```python
from build123d import *

# Parameters (mm, degrees)
BOSS_EXTRUDE1_DEPTH = 10
SKETCH2_R           = 1.5
BOSS_EXTRUDE2_DEPTH = 8


with BuildPart() as part:
    # Sketch1 → Boss-Extrude1 (new body)
    with BuildSketch(Plane(origin=(0, 0, 0), x_dir=(1, 0, 0), z_dir=(0, 1, 0))):
        Polygon((3.175426481, 0), (1.58771324, 2.75), (-1.58771324, 2.75), (-3.175426481, 0), (-1.58771324, -2.75), (1.58771324, -2.75), align=None)
    extrude(amount=-BOSS_EXTRUDE1_DEPTH)

    # Sketch2 → Boss-Extrude2 (add)
    with BuildSketch(Plane(origin=(0, 0, 0), x_dir=(1, 0, 0), z_dir=(0, 1, 0))):
        with Locations(Location((0, 0, 0), (0, 0, 270))):
            Circle(SKETCH2_R)
    extrude(amount=BOSS_EXTRUDE2_DEPTH)


solid = part.part
```
Input: part model. Units: mm. Frame: model coordinates. A direction names the side the tool comes from. Coordinates: 2 decimals unless noted, no trailing zeros. Loops run counter-clockwise (first coordinate to the right, second up) from the corner with the lowest first, then second, coordinate; pieces in that order, holes last. Notation, with made-up numbers: (13, 41) - (64, 41) arc R10 ccw to (64, 50) - close; hole circle Ø4 at (61, 63). An arc over 180 degrees is marked (long way). Answer in a Markdown table with one row per item.
(1) Cut plane D-D on y = 6.75. Output: boundary loops of the cut face in (x, z), plus the area to 3 significant figures.
Model answer:
| item | result |
|---|---|
| outline | circle Ø3 at (0, 0) |
| area | 7.07 mm² |
(2) Cut plane A-A on y = -3. Output: boundary loops of the cut face in (x, z), plus the area to 3 significant figures.
Model answer:
| item | result |
|---|---|
| outline | (-3.18, 0) - (-1.59, -2.75) - (1.59, -2.75) - (3.18, 0) - (1.59, 2.75) - (-1.59, 2.75) - close |
| area | 26.2 mm² |
(3) Cut plane B-B on x = 0. Output: boundary loops of the cut face in (y, z).
Model answer:
| item | result |
|---|---|
| outline | (-10, -2.75) - (0, -2.75) - (0, -1.5) - (8, -1.5) - (8, 1.5) - (0, 1.5) - (0, 2.75) - (-10, 2.75) - close |
(4) Pin query (flat end, axial travel): P1, Ø1, axis at y = -3, z = 1, coming from the -X side; P2, Ø1.5, axis at y = 4.5, z = 0.5, coming from the -X side. Return the tip coordinate at first contact, or that it passes through.
Model answer:
| item | result |
|---|---|
| P1 | stops at x = -2.89 |
| P2 | stops at x = -1.5 |
(5) Set-up query: faces 1 (the face through (0, -5, -2.75)), 2 (the face through (0.45, 3.94, 1.43)). Return all of +Z, -Z, +X, -X, +Y, -Y with unobstructed straight access to the full face (end or side cutting, diameter ignored); none if empty.
Model answer:
| item | result |
|---|---|
| face 1 | -Z, +X, -X, +Y, -Y |
| face 2 | +Y |
(6) Material intervals for L1, parallel to Y at x = 1, z = -2.35; L2, parallel to X at y = 4.25, z = 0.05; L3, parallel to Z at x = -0.75, y = 4, sorted ascending. Write a range as from..to.
Model answer:
| item | result |
|---|---|
| L1 | y = -10..0 |
| L2 | x = -1.5..1.5 |
| L3 | z = -1.3..1.3 |
(7) Cut plane C-C on z = -0.25. Output: boundary loops of the cut face in (x, y), plus the area to 3 significant figures.
Model answer:
| item | result |
|---|---|
| outline | (-3.03, -10) - (3.03, -10) - (3.03, 0) - (1.48, 0) - (1.48, 8) - (-1.48, 8) - (-1.48, 0) - (-3.03, 0) - close |
| area | 84.3 mm² |
